Could you check a few things on this model? Use its own coordinates, in mm. Face numbers are marked on the shaded views. A direction names the side the tool comes from. Round coordinates to 2 decimals unless told otherwise and drop trailing zeros. Write each loop counter-clockwise with the first axis right and the second up, starting at its lowest first coordinate (ties: lowest second). Pieces come first, ordered by that corner, then holes. Notation, with made-up numbers: (81.5, 33.25) -> (127.5, 33.25) arc R8 ccw to (127.5, 48.25) -> close; hole circle Ø8 at (65, 76.25). An arc over 180 degrees is marked (long way). One line per question, with ' | ' between items. Start each with the question number.
1. Imagine slicing it at A-A, the plane z = 5. List the corners of the cut face in (x, y) for me, and give its area (3 significant figures).
2. Imagine slicing it at D-D, the plane z = 0. State how many separate pieces and enclosed holes the cut face has, and give its area (3 significant figures).
3. Thinking about a two-plate mould opening in Z: for the marked faces 1, 2 and 3, which applies, released by +Z, released by -Z, zero draft, split by the parting line, or undercut?
4. If I drill on line 1 along Y through (x, z) = (0, -7.05); line 2 along Y through (x, z) = (6.9, 0); line 3 along Z through (x, y) = (1.75, 112.5), over which ranges is the centre line in solid material (lowest first)? Write a range as [from, to].
5. Imagine slicing it at C-C, the plane y = 52. List the corners of the cut face in (x, z) for me.
6. For the marked faces 4 and 5, which set-ups out of +Z, -Z, +X, -X, +Y, -Y let a thin tool reach every point of the face, with its end or its side?
7. Imagine slicing it at B-B, the plane x = -2.75. List the corners of the cut face in (y, z) for me, and give its area (3 significant figures).
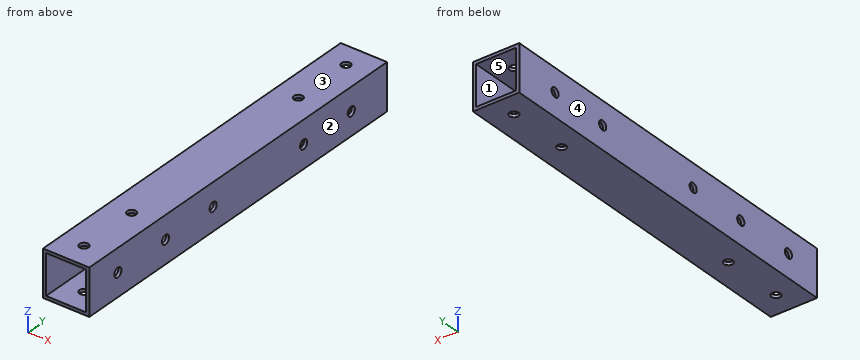
from build123d import *

# Parameters (mm, degrees)
SKETCH_1_W          = 15
SKETCH_1_H          = 15
SKETCH_1_W_2        = 13
SKETCH_1_H_2        = 13
EXTRUDE_1_DEPTH     = 125
SKETCH_2_R          = 1.45
CUT_EXTRUDE_1_DEPTH = 127.119982556
SKETCH_3_R          = 1.5
CUT_EXTRUDE_2_DEPTH = 127.119982556


with BuildPart() as part:
    # 草图1 → 拉伸-薄壁1 (new body)
    with BuildSketch(Plane(origin=(0, 0, 0), x_dir=(1, 0, 0), z_dir=(0, 1, 0))):
        Rectangle(SKETCH_1_W, SKETCH_1_H)
        Rectangle(SKETCH_1_W_2, SKETCH_1_H_2, mode=Mode.SUBTRACT)
    extrude(amount=EXTRUDE_1_DEPTH)

    # 草图2 → 切除-拉伸1 (cut, through all)
    with BuildSketch(Plane.XY.offset(7.5)):
        with Locations((0, 7.5)):
            Circle(SKETCH_2_R)
        with Locations((0, 27.5)):
            Circle(SKETCH_2_R)
        with Locations(Location((0, 97.5, 0), (0, 0, 180))):
            Circle(SKETCH_2_R)
        with Locations(Location((0, 117.5, 0), (0, 0, 180))):
            Circle(SKETCH_2_R)
    extrude(amount=-CUT_EXTRUDE_1_DEPTH, mode=Mode.SUBTRACT)

    # 草图3 → 切除-拉伸2 (cut, through all)
    with BuildSketch(Plane(origin=(7.5, 0, 0), x_dir=(0, 0, -1), z_dir=(1, 0, 0))):
        with Locations((0, 32)):
            Circle(SKETCH_3_R)
        with Locations((0, 12)):
            Circle(SKETCH_3_R)
        with Locations((0, 52)):
            Circle(SKETCH_3_R)
        with Locations((0, 110)):
            Circle(SKETCH_3_R)
        with Locations((0, 90)):
            Circle(SKETCH_3_R)
    extrude(amount=-CUT_EXTRUDE_2_DEPTH, mode=Mode.SUBTRACT)


solid = part.part
Geometry results:
1) outline: (-7.5, 0) -> (-6.5, 0) -> (-6.5, 125) -> (-7.5, 125) -> close; (6.5, 0) -> (7.5, 0) -> (7.5, 125) -> (6.5, 125) -> close | area: 250 mm2
2) separate pieces: 12 | enclosed holes: 0 | area: 220 mm2
3) face 1: undercut | face 2: zero draft | face 3: released by +Z
4) line 1: y = [0, 6.05], [8.95, 26.05], [28.95, 96.05], [98.95, 116.05], [118.95, 125] | line 2: y = [0, 10.5], [13.5, 30.5], [33.5, 50.5], [53.5, 88.5], [91.5, 108.5], [111.5, 125] | line 3: z = [-7.5, -6.5], [6.5, 7.5]
5) outline: (-7.5, -7.5) -> (7.5, -7.5) -> (7.5, -1.5) -> (6.5, -1.5) -> (6.5, -6.5) -> (-6.5, -6.5) -> (-6.5, -1.5) -> (-7.5, -1.5) -> close; (-7.5, 1.5) -> (-6.5, 1.5) -> (-6.5, 6.5) -> (6.5, 6.5) -> (6.5, 1.5) -> (7.5, 1.5) -> (7.5, 7.5) -> (-7.5, 7.5) -> close
6) face 4: +Z, -Z, -X, +Y, -Y | face 5: +Y, -Y
7) outline: (0, -7.5) -> (125, -7.5) -> (125, -6.5) -> (0, -6.5) -> close; (0, 6.5) -> (125, 6.5) -> (125, 7.5) -> (0, 7.5) -> close | area: 250 mm2
